from build123d import *

# Parameters (mm, degrees)
BARRER1_PROFILE_R       = 16
CROQUIS14_W             = 22
CROQUIS14_H             = 30
CROQUIS14_R             = 5.5
SALIENTE_EXTRUIR1_DEPTH = 3
CROQUIS15_R             = 10.841108792
SALIENTE_EXTRUIR2_DEPTH = 19
REDONDEO1_R             = 10


with BuildPart() as part:
    # Barrer1: sweep along a curve in space
    with BuildLine() as barrer1_path:
        Line((-975.305963879, -247.418485436, 3234.31), (-975.305963879, -277.482733156, 3234.31))
        ThreePointArc((-975.305963879, -277.482733156, 3234.31), (-975.305963879, -291.434368594, 3232.3240799), (-975.305963879, -304.277730703, 3226.524074744))
        Line((-975.305963879, -304.277730703, 3226.524074744), (-975.305963879, -390.490454439, 3171.801337481))
        ThreePointArc((-975.305963879, -390.490454439, 3171.801337481), (-975.305963879, -426.451868342, 3155.561323045), (-975.305963879, -465.51644757, 3150.000746764))
        Line((-975.305963879, -465.51644757, 3150.000746764), (-975.305963879, -1014.035511618, 3150.000746764))
        ThreePointArc((-975.305963879, -1144.035511618, 3020.000746764), (-975.305963879, -1105.959393172, 3111.924628318), (-975.305963879, -1014.035511618, 3150.000746764))
        Line((-975.305963879, -1144.035511618, 3020.000746764), (-975.305963879, -1144.035511618, 1960.497178493))
    # Barrer1 profile (on start of the path) → Barrer1 (sweep)
    with BuildSketch(Plane(origin=(-975.305963879, -247.418485436, 3234.31), x_dir=(0, 0, -1), z_dir=(0, -1, 0))):
        Circle(BARRER1_PROFILE_R)
    sweep(path=barrer1_path.line)



with BuildPart() as body_2:
    # Croquis14 → Saliente-Extruir1 (new body)
    with BuildSketch(Plane.XY.offset(3234.31)):
        with Locations((-975.305963879, -216.330473188)):
            Rectangle(CROQUIS14_W, CROQUIS14_H)
        with Locations((-975.305963879, -210.525068536)):
            Circle(CROQUIS14_R, mode=Mode.SUBTRACT)
    extrude(amount=SALIENTE_EXTRUIR1_DEPTH)


with BuildPart() as part_1:
    add(part.part)

    add(body_2.part)  # Saliente-Extruir2 merges body 2
    # Croquis15 → Saliente-Extruir2 (add)
    with BuildSketch(Plane(origin=(0, -247.418485436, 0), x_dir=(1, 0, 0), z_dir=(0, 1, 0))):
        with Locations(Location((-975.305963879, -3234.31, 0), (0, 0, 180))):
            Circle(CROQUIS15_R)
    extrude(amount=SALIENTE_EXTRUIR2_DEPTH)

    # Redondeo1
    # the kernel refuses this fillet: 10 mm, written as the material it takes off along each edge
    with BuildSketch(Plane(origin=(-975.305963879, -247.418485436, 3234.31), x_dir=(0, 0, -1), z_dir=(-1, 0, 0))) as redondeo1_piece_1:
        with BuildLine():
            CenterArc((6, 8.75006661), REDONDEO1_R, 298.954236043, 61.045763957)
            Line((10.841108792, 0), (10.937930967, -0.175001332))
            ThreePointArc((10.937930967, -0.175001332), (13.420554396, -0.2), (16, -0.2))
            Line((16, -0.2), (16.2, 0))
            Line((16.2, 0), (16.2, 8.75006661))
            Line((16.2, 8.75006661), (16, 8.75006661))
        make_face()
    revolve(axis=Axis((-975.305963879, -247.418485436, 3234.31), (0, -1, 0)), mode=Mode.SUBTRACT)


solid = part_1.part
Source: CAD feature listing. Evaluate the final solid. Frame: model axes, mm. A direction names the side the tool comes from. Coordinates: 2 decimals unless noted, no trailing zeros. Order: outer loops, then holes, each group sorted by start corner. A loop starts at its lowest first (then second) coordinate and runs counter-clockwise, first axis right, second up. Notation, with made-up numbers: M 36.5,27 L 71.5,27 A16 ccw 71.5,42 Z; hole C -15,76 d5. An arc over 180 degrees is marked long. Write each question's results on one line, items separated by ' | '. Start each with the question number.
Item 1: Cut plane B-B (z = 2987.5). Return loops of the section in (x, y), and give its area (3 significant figures).
Item 2: First-contact query: pin 1 Ø0.9 at (y, z) = (-213.5, 3235.5) entering from -X; pin 2 Ø3.5 at (y, z) = (-213, 3235.5) entering from +X; pin 3 Ø2 at (x, z) = (-968.5, 2249) entering from +Y. Flat tips, straight axial feed; report the tip coordinate or a pass-through.
Item 3: Draft query along X for faces 1 (the face through (-964.49, -266.97, 3246.1)), 2 (the face through (-975, -1144, 1960.497)). Return one class per face: pulls with the +X half, pulls with the -X half, needs draft (parallel to the pull), parting line crosses it, or undercut.
Item 4: Set-up query: faces 3 (the face through (-970.5, -743.62, 3134.74)), 4 (the face through (-974.6, -1160.02, 2482.83)). Return all of +Z, -Z, +X, -X, +Y, -Y with unobstructed straight access to the full face (end or side cutting, diameter ignored); none if empty.
Item 5: Line query: probe 1 along Y at (x, z) = (-975, 2282); probe 2 along Y at (x, z) = (-976, 2748.5); probe 3 along Z at (x, y) = (-973, -241). Output: solid intervals per line, ascending.
Item 6: Cut plane A-A (y = -675.5). Return loops of the section in (x, z).
Checked values:
1) outline: C -975.31,-1144.04 d32 | area: 804 mm2
2) pin 1: stops at x = -986.31 | pin 2: stops at x = -964.31 | pin 3: stops at y = -1129.13
3) face 1: parting line crosses it | face 2: needs draft
4) face 3: none | face 4: -Z
5) probe 1: y = -1160.03 to -1128.04 | probe 2: y = -1160.02 to -1128.05 | probe 3: z = 3223.72 to 3244.9
6) outline: C -975.31,3150 d32
